Read the model definition and answer for the solid it produces. Units are mm, in the model's axes. A direction names the side the tool comes from. Coordinates: 2 decimals unless noted, no trailing zeros. Write each loop counter-clockwise with the first axis right and the second up, starting at its lowest first coordinate (ties: lowest second). Pieces come first, ordered by that corner, then holes. Notation, with made-up numbers: (46.25, -19) -> (96.25, -19) arc R8 ccw to (96.25, -10) -> close; hole circle Ø4 at (32.5, -25). An arc over 180 degrees is marked (long way). Return JSON: item names as keys, results as strings.
from build123d import *

# Parameters (mm, degrees)
SKETCH1_W                      = 160
SKETCH1_H                      = 160
BOSS_EXTRUDE1_DEPTH            = 70
SKETCH2_W                      = 40
SKETCH2_H                      = 40
CUT_EXTRUDE1_DEPTH             = 134.041346957
SKETCH3_W                      = 80
SKETCH3_H                      = 20
SKETCH3_W_2                    = 20
SKETCH3_H_2                    = 80
CUT_EXTRUDE2_DEPTH             = 60
CUT_EXTRUDE3_REACH             = 135.041
SKETCH4_R                      = 25
M6_CLEARANCE_HOLE1_D           = 6.6
M6_CLEARANCE_HOLE1_CSINK_D     = 6.65
M6_CLEARANCE_HOLE1_CSINK_ANGLE = 100


with BuildPart() as part:
    # Sketch1 → Boss-Extrude1 (new body)
    with BuildSketch(Plane(origin=(0, 0, 0), x_dir=(1, 0, 0), z_dir=(0, 1, 0))):
        Rectangle(SKETCH1_W, SKETCH1_H)
    extrude(amount=BOSS_EXTRUDE1_DEPTH)

    # Sketch2 → Cut-Extrude1 (cut, through all)
    with BuildSketch(Plane(origin=(0, 70, 0), x_dir=(1, 0, 0), z_dir=(0, 1, 0))):
        with Locations((-60, 60)):
            Rectangle(SKETCH2_W, SKETCH2_H)
        with Locations((60, 60)):
            Rectangle(SKETCH2_W, SKETCH2_H)
        with Locations((-60, -60)):
            Rectangle(SKETCH2_W, SKETCH2_H)
        with Locations((60, -60)):
            Rectangle(SKETCH2_W, SKETCH2_H)
    extrude(amount=-CUT_EXTRUDE1_DEPTH, mode=Mode.SUBTRACT)

    # Sketch3 → Cut-Extrude2 (cut)
    with BuildSketch(Plane(origin=(0, 70, 0), x_dir=(1, 0, 0), z_dir=(0, 1, 0))):
        with Locations((0, 70)):
            Rectangle(SKETCH3_W, SKETCH3_H)
        with Locations((-70, 0)):
            Rectangle(SKETCH3_W_2, SKETCH3_H_2)
        with Locations((70, 0)):
            Rectangle(SKETCH3_W_2, SKETCH3_H_2)
        with Locations((0, -70)):
            Rectangle(SKETCH3_W, SKETCH3_H)
    extrude(amount=-CUT_EXTRUDE2_DEPTH, mode=Mode.SUBTRACT)

    # Sketch4 → Cut-Extrude3 (cut, up to next)
    with BuildSketch(Plane(origin=(0, 70, 0), x_dir=(1, 0, 0), z_dir=(0, 1, 0)), mode=Mode.PRIVATE) as cut_extrude3_sk1:
        with Locations(Location((0, 0, 0), (0, 0, 270))):
            Circle(SKETCH4_R)
    cut_extrude3_tool1 = extrude(cut_extrude3_sk1.sketch, amount=-CUT_EXTRUDE3_REACH, mode=Mode.PRIVATE) & part.part
    add(cut_extrude3_tool1.solids().sort_by_distance((0, 70, 0))[0], mode=Mode.SUBTRACT)

    # M6 Clearance Hole1 (through all)
    with Locations(Plane(origin=(0, 10, 0), x_dir=(1, 0, 0), z_dir=(0, 1, 0))):
        with Locations((-70, 25), (-70, -25), (-25, 70), (25, 70), (70, 25), (70, -25), (25, -70), (-25, -70)):
            CounterSinkHole(M6_CLEARANCE_HOLE1_D / 2, M6_CLEARANCE_HOLE1_CSINK_D / 2, counter_sink_angle=M6_CLEARANCE_HOLE1_CSINK_ANGLE)


solid = part.part
1. The part is cut by section D-D (x = 0). Determine the outline of the cut face in (y, z).
Taken from the geometry:
{"outline": "(0, -80) -> (10, -80) -> (10, -60) -> (70, -60) -> (70, -25) -> (0, -25) -> close; (0, 25) -> (70, 25) -> (70, 60) -> (10, 60) -> (10, 80) -> (0, 80) -> close"}
2. The part is cut by section A-A (z = 0). Determine the outline of the cut face in (x, y), then the cut area to 3 significant figures.
Taken from the geometry:
{"outline": "(-80, 0) -> (-25, 0) -> (-25, 70) -> (-60, 70) -> (-60, 10) -> (-80, 10) -> close; (25, 0) -> (80, 0) -> (80, 10) -> (60, 10) -> (60, 70) -> (25, 70) -> close", "area": "5,300 mm2"}
3. Consider L1, parallel to X at y = 7.5, z = 70; L2, parallel to X at y = 37, z = 0. Determine where each line is inside the solid, lowest interval first.
Taken from the geometry:
{"L1": "x = -40 to -28.3, -21.7 to 21.7, 28.3 to 40", "L2": "x = -60 to -25, 25 to 60"}
4. Flat-ended cylindrical pins translate along their axes: pin 1 Ø1 at (x, y) = (-11, 53.5) entering from +Z; pin 2 Ø3 at (x, z) = (3, -22.5) entering from -Y; pin 3 Ø22 at (x, z) = (3.5, 73) entering from +Y; pin 4 Ø12 at (y, z) = (38.5, 55.5) entering from -X. Find the tip coordinate at first contact, or state that the pin passes through.
Taken from the geometry:
{"pin 1": "stops at z = 60", "pin 2": "passes through", "pin 3": "stops at y = 10", "pin 4": "stops at x = -40"}
5. The part is cut by section B-B (y = 22). Determine the outline of the cut face in (x, z), then the cut area to 3 significant figures.
Taken from the geometry:
{"outline": "(-60, -40) -> (-40, -40) -> (-40, -60) -> (40, -60) -> (40, -40) -> (60, -40) -> (60, 40) -> (40, 40) -> (40, 60) -> (-40, 60) -> (-40, 40) -> (-60, 40) -> close; hole circle Ø50 at (0, 0)", "area": "10,800 mm2"}
6. For a pull along Z with two mould halves and no side action, classify faces 1 (the face through (-1, 40, -60)), 2 (the face through (-60, 40, 1)), 3 (the face through (72.619, 4.92, -22.992)) as +Z half, -Z half, draft (parallel to the pull), parting line (faces both ways), or undercut.
Taken from the geometry:
{"face 1": "-Z half", "face 2": "draft", "face 3": "undercut"}
7. The part is cut by section C-C (x = 70). Determine the outline of the cut face in (y, z) (3 decimals), then the cut area to 3 significant figures.
Taken from the geometry:
{"outline": "(0, -40) -> (10, -40) -> (10, -28.325) -> (9.979, -28.3) -> (0, -28.3) -> close; (0, -21.7) -> (9.979, -21.7) -> (10, -21.675) -> (10, 21.675) -> (9.979, 21.7) -> (0, 21.7) -> close; (0, 28.3) -> (9.979, 28.3) -> (10, 28.325) -> (10, 40) -> (0, 40) -> close", "area": "668 mm2"}
8. A tool of negligible diameter and unlimited length cuts with its end or side. For faces 4 (the face through (60, 40, 1)), 5 (the face through (40, 35, -51)), 6 (the face through (-51, 35, 40)), from which of +Z, -Z, +X, -X, +Y, -Y can it reach the whole face along a straight path? Write none if from no direction.
Taken from the geometry:
{"face 4": "+Z, -Z, +X, +Y", "face 5": "-Z, +X, +Y, -Y", "face 6": "+Z, -X, +Y, -Y"}
